Can you work these out from the drawing? Everything is in mm from the part's minimum corner. A direction names the side the tool comes from. Coordinates: 2 decimals unless noted, no trailing zeros. Order: outer loops, then holes, each group sorted by start corner. A loop starts at its lowest first (then second) coordinate and runs counter-clockwise, first axis right, second up. Notation, with made-up numbers: M 26.25,3 L 79.25,3 A22 ccw 79.25,36 Z; hole C 72.5,26 d6. An arc over 180 degrees is marked long. Answer as a JSON object with one key per item and string values.
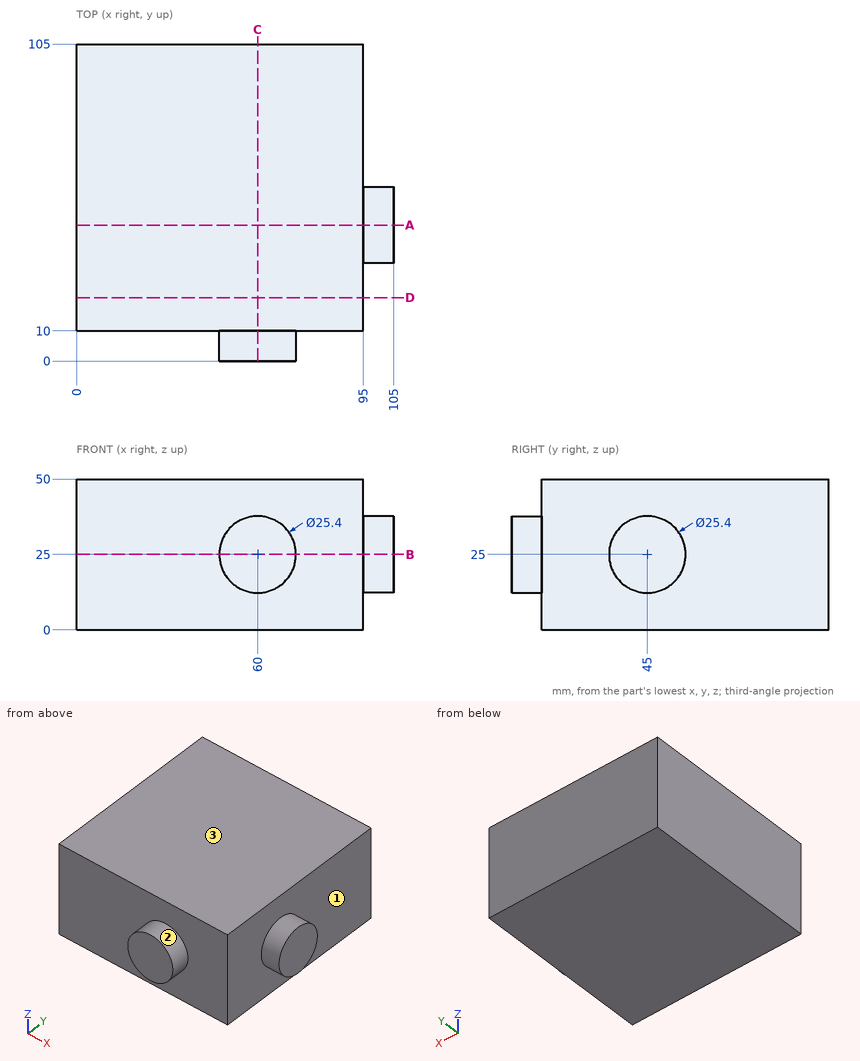
Item 1: I'm going to push a flat-ended pin straight in: pin 1 (2 mm diameter, centred on y = 92.5, z = 29.5, fed in from +X). Where does the tip first touch, or does it pass through?
Answers follow:
{"pin 1": "stops at x = 95"}
Item 2: Please list where these lines run through material, in increasing order: line 1 (X direction, y = 19, z = 27); line 2 (Y direction, x = 7, z = 38); line 3 (X direction, y = 6, z = 32.5).
Answers follow:
{"line 1": "x = 0 to 95", "line 2": "y = 10 to 105", "line 3": "x = 49.75 to 70.25"}
Item 3: I want a section at D-D, the plane y = 21. Write out the boundary of the cut face in (x, z), plus the area to 3 significant figures.
Answers follow:
{"outline": "M 0,0 L 95,0 L 95,50 L 0,50 Z", "area": "4,750 mm^2"}
Item 4: I want a section at A-A, the plane y = 45. Write out the boundary of the cut face in (x, z), plus the area to 3 significant figures.
Answers follow:
{"outline": "M 0,0 L 95,0 L 95,12.3 L 105,12.3 L 105,37.7 L 95,37.7 L 95,50 L 0,50 Z", "area": "5,000 mm^2"}
Item 5: I want a section at B-B, the plane z = 25. Write out the boundary of the cut face in (x, y).
Answers follow:
{"outline": "M 0,10 L 47.3,10 L 47.3,0 L 72.7,0 L 72.7,10 L 95,10 L 95,32.3 L 105,32.3 L 105,57.7 L 95,57.7 L 95,105 L 0,105 Z"}
Item 6: Which directions (+Z, -Z, +X, -X, +Y, -Y) give clear straight access to the entire face, cutting with the end or side of a thin tool? Please do the marked faces 1, 2 and 3.
Answers follow:
{"face 1": "+X", "face 2": "-Y", "face 3": "+Z, +X, -X, +Y, -Y"}
Item 7: I want a section at C-C, the plane x = 60. Write out the boundary of the cut face in (y, z), plus the area to 3 significant figures.
Answers follow:
{"outline": "M 0,12.3 L 10,12.3 L 10,0 L 105,0 L 105,50 L 10,50 L 10,37.7 L 0,37.7 Z", "area": "5,000 mm^2"}
